The model under review builds one solid part; all positions refer to its coordinate system, in mm. A direction names the side the tool comes from. Give positions to 0.01 mm unless a question says otherwise; leave off trailing zeros. Order: outer loops, then holes, each group sorted by start corner. A loop starts at its lowest first (then second) coordinate and runs counter-clockwise, first axis right, second up. Notation, with made-up numbers: (-40, 76.5) - (-30, 76.5) arc R22 ccw to (-30, 106.5) - close; hole circle Ø10 at (45, 48.25). An arc over 180 degrees is marked (long way). Use CSV: the item, a comma, the result in double quotes.
```python
from build123d import *

# Parameters (mm, degrees)
BOSS_EXTRUDE1_DEPTH = 1
SKETCH2_W           = 14
SKETCH2_H           = 14
CUT_EXTRUDE1_DEPTH  = 112.007775968
CUT_EXTRUDE2_DEPTH  = 112.007775968


with BuildPart() as part:
    # Sketch1 → Boss-Extrude1 (new body)
    with BuildSketch(Plane(origin=(0, 0, 0), x_dir=(1, 0, 0), z_dir=(0, 1, 0))):
        Polygon((-16.174938897, 86.307472271), (69.805061103, 86.307472271), (38.792758309, -44.321715415), (10.792758309, -44.321715415), (42.145061103, 63.898255059), (-16.174938897, 64.637472271), align=None)
    extrude(amount=BOSS_EXTRUDE1_DEPTH)

    # Sketch2 → Cut-Extrude1 (cut, through all)
    with BuildSketch(Plane(origin=(0, 0, 0), x_dir=(1, 0, 0), z_dir=(0, 1, 0))):
        with Locations((-6.014238297, 75.907608588)):
            Rectangle(SKETCH2_W, SKETCH2_H)
        with Locations((27.168678058, 75.880355848)):
            Rectangle(SKETCH2_W, SKETCH2_H)
        Polygon((47.235283442, 69.379844428), (61.104296679, 67.469223626), (65.705307468, 80.691579684), (51.836294232, 82.602200486), align=None)
    extrude(amount=CUT_EXTRUDE1_DEPTH, mode=Mode.SUBTRACT)

    # Sketch3 → Cut-Extrude2 (cut, through all)
    with BuildSketch(Plane(origin=(0, 1, 0), x_dir=(1, 0, 0), z_dir=(0, 1, 0))):
        Polygon((42.039756476, 48.29086531), (55.808834799, 45.758577387), (53.276546876, 31.989499063), (39.507468553, 34.521786986), align=None)
        Polygon((46.302698973, 11.55658303), (43.259967448, -2.108766759), (29.594617659, 0.933964766), (32.637349184, 14.599314555), align=None)
        Polygon((38.601429809, -20.915974937), (35.546831549, -34.578677066), (21.88412942, -31.524078805), (24.93872768, -17.861376676), align=None)
    extrude(amount=-CUT_EXTRUDE2_DEPTH, mode=Mode.SUBTRACT)


solid = part.part
```
Item 1: Take a section at C-C, the plane z = -76.5. Give the boundary of the cut face in (x, y).
Results list:
outline,"(-16.17, 0) - (-13.01, 0) - (-13.01, 1) - (-16.17, 1) - close; (0.99, 0) - (20.17, 0) - (20.17, 1) - (0.99, 1) - close; (34.17, 0) - (49.71, 0) - (49.71, 1) - (34.17, 1) - close; (64.25, 0) - (67.48, 0) - (67.48, 1) - (64.25, 1) - close"
Item 2: Take a section at A-A, the plane x = -9. Give the boundary of the cut face in (y, z).
Results list:
outline,"(0, -86.31) - (1, -86.31) - (1, -82.91) - (0, -82.91) - close; (0, -68.91) - (1, -68.91) - (1, -64.55) - (0, -64.55) - close"
Item 3: Clearance check with a flat-ended pin moving along its axis: pin 1 (5 mm diameter, centred on x = 22, z = -70.5, fed in from +Y). State where the tip first meets the part, or that it passes through.
Results list:
pin 1,"stops at y = 1"
Item 4: Take a section at B-B, the plane y = 0.2. State how many separate pieces and enclosed holes the cut face has, and give its area (3 significant figures).
Results list:
separate pieces,"1"
enclosed holes,"6"
area,"3,400 mm2"
Item 5: Take a section at D-D, the plane z = 24.5. Give the boundary of the cut face in (x, y).
Results list:
outline,"(16.54, 0) - (23.45, 0) - (23.45, 1) - (16.54, 1) - close; (37.8, 0) - (43.5, 0) - (43.5, 1) - (37.8, 1) - close"
Item 6: Mouldability with a two-part tool opening along X and no side actions: class faces 3 (the face through (26.25, 0.49, -9.03)), 4 (the face through (54.516, 0.493, -21.907)), 5 (the face through (46.488, 0.507, -33.238)), 6 (the face through (36.52, 0.51, 0.61)) as pulls with the +X half, pulls with the -X half, needs draft (parallel to the pull), parting line crosses it, or undercut.
Results list:
face 3,"pulls with the -X half"
face 4,"pulls with the +X half"
face 5,"undercut"
face 6,"undercut"
Item 7: Tool access review of faces 1 (the face through (28.811, 0.507, 33.073)), 2 (the face through (33, 1, -31)): name each direction out of +Z, -Z, +X, -X, +Y, -Y from which nothing blocks a thin tool from reaching the whole face with its end or side.
Results list:
face 1,"+Y, -Y"
face 2,"+Z, -Z, +X, -X, +Y"
Item 8: Wall thickness on L1, parallel to X at y = 0.5, z = -10.5; L2, parallel to X at y = 0.95, z = -80.5; L3, parallel to X at y = 0.35, z = -8.5: over which ranges is each line inside the solid? List them lowest first.
Results list:
L1,"x = 26.68 to 31.72, 46.07 to 51.81"
L2,"x = -16.17 to -13.01, 0.99 to 20.17, 34.17 to 51.1, 65.64 to 68.43"
L3,"x = 26.1 to 31.28, 45.62 to 51.33"
